For this review, take the finished solid that the model builds, in its own axes (mm). Face numbers are marked on the shaded views. A direction names the side the tool comes from. Round coordinates to 2 decimals unless told otherwise and drop trailing zeros. Order: outer loops, then holes, each group sorted by start corner. A loop starts at its lowest first (then second) coordinate and runs counter-clockwise, first axis right, second up. Notation, with made-up numbers: M -26,-28 L -17,-28 A22 cw -17,7 Z; hole C 26,80 d8. An arc over 180 degrees is marked long. Use a Markdown table: item, result.
from build123d import *

# Parameters (mm, degrees)
P_IDAT_VYSUNUT_M1_DEPTH  = 25
SKICA2_R                 = 2
ODEBRAT_VYSUNUT_M1_DEPTH = 2.01
ZAOBLIT1_R               = 1
ZKOSEN_4_SIZE            = 0.25
ZKOSEN_5_SIZE            = 0.5
ZKOSEN_6_SIZE            = 0.5


with BuildPart() as part:
    # Skica1 → Přidat vysunutím1 (new body)
    with BuildSketch(Plane.XY):
        Polygon((0, 0), (0, 8), (35, 8), (35, 0), (35, -4.21), (25.3, -4.21), (25.3, 0), (23.546281771, 2.09), (23.546281771, 2.7), (25.3, 4.79), (25.3, 5.74), (25.05, 5.99), (9.95, 5.99), (9.7, 5.74), (9.7, 4.79), (11.453718229, 2.7), (11.453718229, 2.09), (9.7, 0), (9.7, -4.21), (0, -4.21), align=None)
    extrude(amount=P_IDAT_VYSUNUT_M1_DEPTH)

    # Skica2 → Odebrat vysunutím1 (cut)
    with BuildSketch(Plane(origin=(0, 8, 0), x_dir=(1, 0, 0), z_dir=(0, 1, 0))):
        with Locations(Location((17.5, -18, 0), (0, 0, 180))):
            Circle(SKICA2_R)
    extrude(amount=-ODEBRAT_VYSUNUT_M1_DEPTH, mode=Mode.SUBTRACT)

    # Zaoblit1
    zaoblit1_edges = [part.edges().sort_by_distance(p)[0] for p in [
        (0, 1.895, 0),
        (35, 1.895, 0),
        (0, 1.895, 25),
        (35, 1.895, 25),
    ]]
    fillet(zaoblit1_edges, radius=ZAOBLIT1_R)

    # Zkosení4
    zkosen_4_edges = [part.edges().sort_by_distance(p)[0] for p in [
        (9.7, -2.105, 25),
        (10.576859115, 1.045, 25),
        (11.453718229, 2.395, 25),
        (25.3, -2.105, 0),
        (24.423140885, 1.045, 0),
        (23.546281771, 2.395, 0),
        (24.423140885, 3.745, 0),
        (25.3, 5.265, 0),
        (25.175, 5.865, 0),
        (17.5, 5.99, 0),
        (9.825, 5.865, 0),
        (9.7, 5.265, 0),
        (10.576859115, 3.745, 25),
        (10.576859115, 3.745, 0),
        (11.453718229, 2.395, 0),
        (10.576859115, 1.045, 0),
        (9.7, -2.105, 0),
        (9.7, 5.265, 25),
        (9.825, 5.865, 25),
        (17.5, 5.99, 25),
        (25.175, 5.865, 25),
        (25.3, 5.265, 25),
        (24.423140885, 3.745, 25),
        (23.546281771, 2.395, 25),
        (24.423140885, 1.045, 25),
        (25.3, -2.105, 25),
    ]]
    chamfer(zkosen_4_edges, length=ZKOSEN_4_SIZE)

    # Zkosení5
    zkosen_5_edges = [part.edges().sort_by_distance(p)[0] for p in [
        (17.5, 8, 25),
        (17.5, 8, 0),
        (0, 8, 12.5),
        (35, 8, 12.5),
        (0.292893219, 8, 24.707106781),
        (0.292893219, 8, 0.292893219),
        (34.707106781, 8, 0.292893219),
        (34.707106781, 8, 24.707106781),
    ]]
    chamfer(zkosen_5_edges, length=ZKOSEN_5_SIZE)

    # Zkosení6
    zkosen_6_edges = [part.edges().sort_by_distance(p)[0] for p in [
        (19.5, 8, 18),
    ]]
    chamfer(zkosen_6_edges, length=ZKOSEN_6_SIZE)


solid = part.part
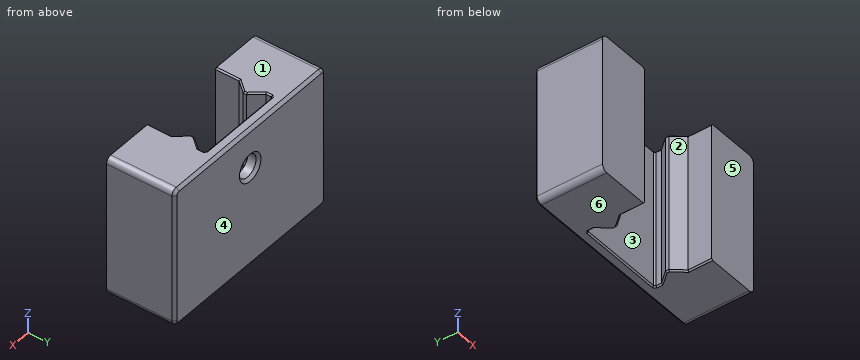
Q1. Add section B-B (z = 18). Write out the cut boundary in (x, y).
Determined:
| item | result |
|---|---|
| outline | M 0,-4.21 L 9.7,-4.21 L 9.7,0 L 11.45,2.09 L 11.45,2.7 L 9.7,4.79 L 9.7,5.74 L 9.95,5.99 L 15.5,5.99 L 15.5,7.5 L 15,8 L 0.5,8 L 0,7.5 Z; M 19.5,5.99 L 25.05,5.99 L 25.3,5.74 L 25.3,4.79 L 23.55,2.7 L 23.55,2.09 L 25.3,0 L 25.3,-4.21 L 35,-4.21 L 35,7.5 L 34.5,8 L 20,8 L 19.5,7.5 Z |
Q2. Clearance check with flat-ended pins moving along their axes: pin 1 (2 mm diameter, centred on x = 18.5, z = 20, fed in from -Y); pin 2 (7.5 mm diameter, centred on x = 20.5, z = 18, fed in from -Y). State where each tip first meets the part, or that it passes through.
Determined:
| item | result |
|---|---|
| pin 1 | stops at y = 5.99 |
| pin 2 | stops at y = 1.25 |
Q3. Machinability: for the marked faces 1 and 2, which of the approach directions +Z, -Z, +X, -X, +Y, -Y give a long, thin tool a straight path to every point of the face, cutting with its end or side? Answer none if there is none.
Determined:
| item | result |
|---|---|
| face 1 | +Z, +X, -X, +Y, -Y |
| face 2 | +Z, -Z, -Y |
Q4. Draft analysis for pull direction Y (two halves, no side actions). For the marked faces 3, 4, 5 and 6, state which applies: pulls with the +Y half, pulls with the -Y half, needs draft (parallel to the pull), parting line crosses it, or undercut.
Determined:
| item | result |
|---|---|
| face 3 | undercut |
| face 4 | pulls with the +Y half |
| face 5 | pulls with the -Y half |
| face 6 | needs draft |
Q5. Add section D-D (x = 22.5). Write out the cut boundary in (y, z).
Determined:
| item | result |
|---|---|
| outline | M 5.99,0.25 L 6.24,0 L 7.5,0 L 8,0.5 L 8,24.5 L 7.5,25 L 6.24,25 L 5.99,24.75 Z |
Q6. Add section C-C (x = 17.5). Write out the cut boundary in (y, z).
Determined:
| item | result |
|---|---|
| outline | M 5.99,0.25 L 6.24,0 L 7.5,0 L 8,0.5 L 8,15.5 L 7.5,16 L 5.99,16 Z; M 5.99,20 L 7.5,20 L 8,20.5 L 8,24.5 L 7.5,25 L 6.24,25 L 5.99,24.75 Z |
Q7. Wall thickness on line 1 along X through (y, z) = (-1, 15.75); line 2 along X through (y, z) = (4.5, 20.5); line 3 along Z through (x, y) = (17.5, 6.75): over which ranges is each line inside the solid? List them lowest first. Write a range as [from, to].
Determined:
| item | result |
|---|---|
| line 1 | x = [0, 9.7], [25.3, 35] |
| line 2 | x = [0, 9.94], [25.06, 35] |
| line 3 | z = [0, 16], [20, 25] |
Q8. Add section A-A (y = -1). Write out the cut boundary in (x, z), then the cut area to 3 significant figures.
Determined:
| item | result |
|---|---|
| outline | M 0,1 A1 ccw 1,0 L 9.45,0 L 9.7,0.25 L 9.7,24.75 L 9.45,25 L 1,25 A1 ccw 0,24 Z; M 25.3,0.25 L 25.55,0 L 34,0 A1 ccw 35,1 L 35,24 A1 ccw 34,25 L 25.55,25 L 25.3,24.75 Z |
| area | 484 mm^2 |
